The listing builds one solid part. Answer for the finished solid, in the listing's coordinates (mm). A direction names the side the tool comes from. Round coordinates to 2 decimals unless told otherwise and drop trailing zeros. Order: outer loops, then holes, each group sorted by start corner. A loop starts at its lowest first (then second) coordinate and runs counter-clockwise, first axis right, second up. Notation, with made-up numbers: (27, 33) - (79, 33) arc R7 cw to (79, 38) - close; hole circle Ø8 at (-3.75, 44.5). An arc over 180 degrees is marked (long way). Use CSV: the item, a comma, the result in double quotes. Start each with the question number.
Item 1: Determine the mould class of faces 1 (the flat face through (209, 142, 0)), 2 (the flat face through (395.13, 19.25, 1.5)) for opening direction X: +X half, -X half, draft (parallel to the pull), parting line (faces both ways), or undercut.
Item 2: Find section A-A, the plane x = 196. Give the vertices of the cut face in (y, z), plus the area to 3 significant figures.
Item 3: Straight lines are drawn through the part: line 1 along Y through (x, z) = (215, 0.85); line 2 along X through (y, z) = (237, 2.6); line 3 along X through (y, z) = (258.5, 0.75). For each, find the intervals that lie inside material, in ascending order. Write a range as [from, to].
Item 4: For faces 3 (the flat face through (209, 142, 2.95)), 4 (the flat face through (434.347, 260.744, 1.496)), determine the directions among +Z, -Z, +X, -X, +Y, -Y from which every point of the face is accessible in a straight line to the end or side of a thin tool.
```python
from build123d import *

# Parameters (mm, degrees)
F0_W     = 2.95
F0_H     = 30
F0_W_2   = 50
F0_H_2   = 2.95
F1_DEPTH = 2.95
F3_D     = 5
F5_DEPTH = 2.95


# Not quite as in the source:
# - a feature names something its author has since deleted; it is built from what else it names


with BuildPart() as f1:
    # F0 (on Top) → F1 (new body)
    with BuildSketch(Plane.XY):
        Polygon((-37.9051826894, 0), (12.0948173106, 0), (462.0948173106, 0), (462.0948173106, 280), (62.0948173106, 280), (-37.9051826894, 280), align=None)
        with Locations((40.9065613726, 32.5)):
            Rectangle(F0_W, F0_H, mode=Mode.SUBTRACT)
        with Locations((59.4315613726, 66.475)):
            Rectangle(F0_W_2, F0_H_2, mode=Mode.SUBTRACT)
        with Locations((209.4315613726, 66.475)):
            Rectangle(F0_W_2, F0_H_2, mode=Mode.SUBTRACT)
        with Locations((359.8315613726, 32.5)):
            Rectangle(F0_W, F0_H, mode=Mode.SUBTRACT)
        with Locations((359.4315613726, 66.475)):
            Rectangle(F0_W_2, F0_H_2, mode=Mode.SUBTRACT)
        with Locations((59.4315613726, 213.525)):
            Rectangle(F0_W_2, F0_H_2, mode=Mode.SUBTRACT)
        with Locations((40.9065613726, 247.5)):
            Rectangle(F0_W, F0_H, mode=Mode.SUBTRACT)
        with Locations((209.4315613726, 213.525)):
            Rectangle(F0_W_2, F0_H_2, mode=Mode.SUBTRACT)
        with Locations((359.4315613726, 213.525)):
            Rectangle(F0_W_2, F0_H_2, mode=Mode.SUBTRACT)
        with Locations((359.8315613726, 247.5)):
            Rectangle(F0_W, F0_H, mode=Mode.SUBTRACT)
    extrude(amount=F1_DEPTH)

    # F3 (through all)
    with Locations(Plane.XY.offset(2.95)):
        with Locations((-27.9051826894, 10), (-27.9051826894, 270), (452.0948173106, 10), (452.0948173106, 270)):
            Hole(F3_D / 2)

    # F4 (on face) → F5 (cut)
    with BuildSketch(Plane.XY.offset(2.95)):
        Polygon((402.1092280247, 232.6776666521), (387.9670924009, 218.5355310284), (390.0530574054, 216.4495660239), (404.1951930292, 230.5917016476), align=None)
        Polygon((441.5175263771, 267.9140349955), (439.4315613726, 270), (425.2894257488, 255.8578643763), (427.3753907533, 253.7718993718), align=None)
        Polygon((386.4580381415, 273.5950192639), (384.372073137, 271.5090542594), (405.5852765726, 250.2958508238), (407.6712415771, 252.3818158283), align=None)
        Polygon((386.4580381415, 6.4049807361), (407.6712415771, 27.6181841717), (405.5852765726, 29.7041491762), (384.372073137, 8.4909457406), align=None)
        Polygon((427.3753907533, 26.2281006282), (425.2894257488, 24.1421356237), (439.4315613726, 10), (441.5175263771, 12.0859650045), align=None)
        Polygon((387.9670924009, 61.4644689716), (402.1092280247, 47.3223333479), (404.1951930292, 49.4082983524), (390.0530574054, 63.5504339761), align=None)
    extrude(amount=-F5_DEPTH, mode=Mode.SUBTRACT)


solid = f1.part
```
Worked out:
1,face 1,"draft"
1,face 2,"undercut"
2,outline,"(0, 0) - (65, 0) - (65, 2.95) - (0, 2.95) - close; (67.95, 0) - (212.05, 0) - (212.05, 2.95) - (67.95, 2.95) - close; (215, 0) - (280, 0) - (280, 2.95) - (215, 2.95) - close"
2,area,"809 mm²"
3,line 1,"y = [0, 65], [67.95, 212.05], [215, 280]"
3,line 2,"x = [-37.91, 39.43], [42.38, 358.36], [361.31, 462.09]"
3,line 3,"x = [-37.91, 39.43], [42.38, 358.36], [361.31, 397.38], [401.55, 427.93], [432.1, 462.09]"
4,face 3,"+Z, +X, -X, +Y, -Y"
4,face 4,"+Z, -Z"
